Autodesk Inventor part; units mm, degrees
ref_plane "YZ Plane" through (0, 0, 0) normal (1, 0, 0) x (0, 1, 0)
ref_plane "XZ Plane" through (0, 0, 0) normal (0, 1, 0) x (-1, 0, 0)
ref_plane "XY Plane" through (0, 0, 0) normal (0, 0, 1) x (1, 0, 0)
sketch "Sketch1" plane through (0, 0, 0) normal (0, 0, 1) x (1, 0, 0)
  circle A0 centre (4, 4) radius 1.2
  circle A1 centre (4, 4) radius 2
  point P0 (0, 0)
  dimension "d0" = 4
extrude "Extrusion1" add sketch "Sketch1" against normal blind 10 contours A0 | A1
sketch "Sketch2" plane through (4, 4, 0) normal (0, 0, 1) x (1, 0, 0)
  circle A0 centre (0, 0) radius 2
  circle A1 centre (0, 0) radius 3.65
  point P0 (-4, -4)
  dimension "d3" = 7.3
extrude "Extrusion2" add sketch "Sketch2" along normal blind 2.3 contours A0 | A1
fillet "Fillet1" radius 2.2 1 edges at (0.35, 4, 2.3)
sketch "Sketch4" plane through (4, 4, 2.3) normal (0, 0, 1) x (1, 0, 0)
  circle A0 centre (0, 0) radius 1.45
  line L0 (0.7217, 1.25) -> (1.4434, 0)
  line L1 (1.4434, 0) -> (0.7217, -1.25)
  line L2 (0.7217, -1.25) -> (-0.7217, -1.25)
  line L3 (-0.7217, -1.25) -> (-1.4434, 0)
  line L4 (-1.4434, 0) -> (-0.7217, 1.25)
  line L5 (-0.7217, 1.25) -> (0.7217, 1.25)
  point P0 (-4, -4)
  dimension "d10" = 2.5
extrude "Extrusion4" cut sketch "Sketch4" along normal mid plane 4 contours L0 L1 L2 L3 L4 L5
thread "Thread1"
properties part number "m3 6" material "Steel"
Geometry check sheet. Reference: the model listing, model coordinates, mm. A direction names the side the tool comes from. Coordinates: 2 decimals unless noted, no trailing zeros. Write each loop counter-clockwise with the first axis right and the second up, starting at its lowest first coordinate (ties: lowest second). Pieces come first, ordered by that corner, then holes. Notation, with made-up numbers: (11, 8) -> (63, 8) arc R11 ccw to (63, 29) -> close; hole circle Ø8 at (-8.5, -29). An arc over 180 degrees is marked (long way). Use CSV: the item, a comma, the result in double quotes. Start each with the question number.
Item 1: Mould release check, pull along Y, two halves, no side actions. Record for faces 3 (the cylindrical face through (2.4, 2.8, -4.9)), 4 (the flat face through (5.088, 3.384, 1.286)), 5 (the flat face through (4, 5.25, 1)), 6 (the flat face through (4, 4, -10)): released by +Y, released by -Y, zero draft, split by the parting line, or undercut.
Item 2: Cross-section at A-A, the plane z = -1. Record the cut outline in (x, y).
Item 3: Thickness scan on line 1 (Y direction, x = 5.25, z = 1.5); line 2 (Y direction, x = 5.25, z = -4.75); line 3 (X direction, y = 3, z = -4.75). Record the ranges inside material, lowest first.
Item 4: Set-up check for faces 1 (the flat face through (6, 2, 0)), 2 (the flat face through (2.912, 4.616, 1.286)): record each of +Z, -Z, +X, -X, +Y, -Y from which the full face is reachable in a straight line by a thin tool's end or side.
Item 5: Depth check by flat-ended pin: pin 1 Ø2 at (y, z) = (2.5, -4.5) entering from -X; pin 2 Ø2 at (x, y) = (1, 3.5) entering from -Z; pin 3 Ø1.2 at (x, z) = (4.5, 1.5) entering from +Y. Enter the tip coordinate at first touch or a pass-through.
Answers:
1,face 3,"split by the parting line"
1,face 4,"undercut"
1,face 5,"undercut"
1,face 6,"zero draft"
2,outline,"circle Ø4 at (4, 4)"
3,line 1,"1.11 to 3.67, 4.33 to 6.89"
3,line 2,"2.44 to 5.56"
3,line 3,"2.27 to 5.73"
4,face 1,"-Z"
4,face 2,"+Z"
5,pin 1,"x = 2.06"
5,pin 2,"z = 0"
5,pin 3,"y = 7.47"
